from build123d import *

# Parameters (mm, degrees)
SWEEP1_PROFILE_R                = 6.5
TAP_DRILL_FOR_M6X1_0_TAP1_D     = 5
TAP_DRILL_FOR_M6X1_0_TAP1_DEPTH = 22
TAP_DRILL_FOR_M6X1_0_TAP1_TIP   = 1.502151548


with BuildPart() as part:
    # Sweep1: sweep along a path in Sketch1
    with BuildLine(Plane(origin=(0, 0, 0), x_dir=(1, 0, 0), z_dir=(0, 1, 0))) as sweep1_path:
        Line((-50, -34), (-50, -13))
        ThreePointArc((-50, -13), (-46.192388155, -3.807611845), (-37, 0))
        Line((-37, 0), (37, 0))
        ThreePointArc((37, 0), (46.192388155, -3.807611845), (50, -13))
        Line((50, -13), (50, -34))
    # Sweep1 profile (on start of the path) → Sweep1 (sweep)
    with BuildSketch(Plane(origin=(-50, 0, 34), x_dir=(-1, 0, 0), z_dir=(0, 0, -1))):
        Circle(SWEEP1_PROFILE_R)
    sweep(path=sweep1_path.line)

    # Tap Drill for M6x1.0 Tap1
    with Locations(Plane.XY.offset(34)):
        with Locations((-50, 0), (50, 0)):
            Hole(TAP_DRILL_FOR_M6X1_0_TAP1_D / 2, depth=TAP_DRILL_FOR_M6X1_0_TAP1_DEPTH)
            with Locations((0, 0, -(TAP_DRILL_FOR_M6X1_0_TAP1_DEPTH + TAP_DRILL_FOR_M6X1_0_TAP1_TIP / 2))):  # 118° drill point
                Cone(0, TAP_DRILL_FOR_M6X1_0_TAP1_D / 2, TAP_DRILL_FOR_M6X1_0_TAP1_TIP, mode=Mode.SUBTRACT)


solid = part.part
Build history of the part. All positions in model axes, mm. A direction names the side the tool comes from. Give positions to 0.01 mm unless a question says otherwise; leave off trailing zeros. Write each loop counter-clockwise with the first axis right and the second up, starting at its lowest first coordinate (ties: lowest second). Pieces come first, ordered by that corner, then holes. Notation, with made-up numbers: (-28, -23.5) - (-9, -23.5) arc R7 cw to (-9, -19.5) - close; hole circle Ø5 at (29.5, 1). An arc over 180 degrees is marked (long way). Use one line per item in the form item = value. Start each with the question number.
1. Band-saw the part on A-A on z = 14. Write the cut outline in (x, y), plus the area to 3 significant figures.
2. Two-plate mould, pull along Y, no slides. Class faces 1 (the face through (47.69, -0.96, 22.85)), 2 (the face through (-49.6, -0.17, 10.76)), 3 (the face through (43.506, 0.286, 23.647)), 4 (the face through (50, -3, 34)): released by +Y, released by -Y, zero draft, split by the parting line, or undercut.
3. Probe line 1 (Y direction, x = -50, z = 21); line 2 (X direction, y = -2.25, z = 15); line 3 (X direction, y = 2, z = 25). List the from-to ranges inside material, lowest first. Write a range as [from, to].
4. Drop flat-ended pins along their axis: pin 1 Ø5 at (y, z) = (-3, 12.5) entering from -X; pin 2 Ø1.5 at (y, z) = (-2.5, 20) entering from -X; pin 3 Ø5 at (y, z) = (-2.5, 2.5) entering from +X; pin 4 Ø3 at (x, y) = (-18.5, 1.5) entering from -Z. Give the stop position or say it passes through.
5. 3-axis set-ups, long thin cutter, end or side, ignore diameter. For faces 5 (the face through (-50, -3, 34)), 6 (the face through (0.518, -3.955, 5.158)), 7 (the face through (-43.506, 0.286, 23.353)): which of +Z, -Z, +X, -X, +Y, -Y reach the whole face in a straight line?
6. Band-saw the part on B-B on y = 4. Write the cut outline in (x, z), plus the area to 3 significant figures.
7. Band-saw the part on C-C on x = -35. Write the cut outline in (y, z), plus the area to 3 significant figures.
Conclusion:
q1.outline = circle Ø13 at (-50, 0); circle Ø13 at (50, 0); hole circle Ø5 at (-50, 0); hole circle Ø5 at (50, 0)
q1.area = 226 mm²
q2.face_1 = undercut
q2.face_2 = undercut
q2.face_3 = split by the parting line
q2.face_4 = zero draft
q3.line_1 = [-6.5, -2.5], [2.5, 6.5]
q3.line_2 = [-56.1, -51.09], [-48.91, -43.9], [43.9, 48.91], [51.09, 56.1]
q3.line_3 = [-56.18, -51.5], [-48.5, -43.82], [43.82, 48.5], [51.5, 56.18]
q4.pin_1 = -56.48
q4.pin_2 = -56.26
q4.pin_3 = 54.5
q4.pin_4 = -6.5
q5.face_5 = +Z, +X, -X, +Y, -Y
q5.face_6 = none
q5.face_7 = +Z
q6.outline = (-55.12, 13) arc R18.12 ccw to (-37, -5.12) - (37, -5.12) arc R18.12 ccw to (55.12, 13) - (55.12, 34) - (44.88, 34) - (44.88, 13) arc R7.88 cw to (37, 5.12) - (-37, 5.12) arc R7.88 cw to (-44.88, 13) - (-44.88, 34) - (-55.12, 34) - close
q6.area = 1,610 mm²
q7.outline = circle Ø13 at (0, 0)
q7.area = 133 mm²
